from build123d import *

# Parameters (mm, degrees)
CYLINDER008_R     = 5.5
CYLINDER008_DEPTH = 20
CYLINDER009_R     = 1.4
CYLINDER009_DEPTH = 20
BOX002_W          = 16
BOX002_H          = 32
BOX002_DEPTH      = 13
FILLET008_R       = 7
FILLET009_R       = 6
FILLET010_R       = 1
FILLET011_R       = 1
CHAMFER007_SIZE   = 1


with BuildPart() as cylinder:
    # Cylinder008 → Cylinder008 (new body)
    with BuildSketch(Plane.XY):
        Circle(CYLINDER008_R)
    extrude(amount=CYLINDER008_DEPTH)


with BuildPart() as fusion004:
    # Cylinder009 → Cylinder009 (new body)
    with BuildSketch(Plane(origin=(-10, 18, 6.5), x_dir=(0, 0, -1), z_dir=(1, 0, 0))):
        Circle(CYLINDER009_R)
    extrude(amount=CYLINDER009_DEPTH)

    # Fusion004: union Cylinder
    add(cylinder.part)


with BuildPart() as obj1:
    # Box002 → Box002 (new body)
    with BuildSketch(Plane(origin=(-8, -8, 0), x_dir=(1, 0, 0), z_dir=(0, 0, 1))):
        with Locations((8, 16)):
            Rectangle(BOX002_W, BOX002_H)
    extrude(amount=BOX002_DEPTH)

    # Fillet008
    fillet008_edges = [obj1.edges().sort_by_distance(p)[0] for p in [
        (-8, -8, 6.5),
        (8, -8, 6.5),
    ]]
    fillet(fillet008_edges, radius=FILLET008_R)

    # Fillet009
    fillet009_edges = [obj1.edges().sort_by_distance(p)[0] for p in [
        (0, 24, 13),
        (0, 24, 0),
    ]]
    fillet(fillet009_edges, radius=FILLET009_R)

    # Fillet010
    fillet010_edges = [obj1.edges().sort_by_distance(p)[0] for p in [
        (8, 8.5, 13),
    ]]
    fillet(fillet010_edges, radius=FILLET010_R)

    # Cut004: cut Fusion004
    add(fusion004.part, mode=Mode.SUBTRACT)

    # Fillet011
    fillet011_edges = [obj1.edges().sort_by_distance(p)[0] for p in [
        (-5.5, 0, 0),
        (-5.5, 0, 13),
    ]]
    fillet(fillet011_edges, radius=FILLET011_R)

    # Chamfer007
    chamfer007_edges = [obj1.edges().sort_by_distance(p)[0] for p in [
        (-8, 18, 7.9),
        (8, 18, 7.9),
    ]]
    chamfer(chamfer007_edges, length=CHAMFER007_SIZE)


solid = obj1.part
Input: part model. Units: mm. Frame: model coordinates. Round coordinates to 2 decimals unless told otherwise and drop trailing zeros. Order: outer loops, then holes, each group sorted by start corner. A loop starts at its lowest first (then second) coordinate and runs counter-clockwise, first axis right, second up.
1. Mould query, pull axis Z, two halves, no side actions, for faces 1 (the face through (0, 11, 0)), 2 (the face through (0.098, 22.289, 11.196)), 3 (the face through (-0.098, 16.633, 6.803)). Classes: released by +Z, released by -Z, zero draft, split by the parting line, or undercut.
The answers:
face 1: released by -Z
face 2: released by +Z
face 3: undercut
2. Pin query (flat end, axial travel): P1, Ø6, axis at x = -5.5, z = 5.5, coming from the -Y side; P2, Ø2, axis at x = 2.5, z = 8.5, coming from the -Y side; P3, Ø1.5, axis at x = -6.5, z = 3, coming from the +Y side. Return the tip coordinate at first contact, or that it passes through.
The answers:
P1: stops at y = -7.84
P2: stops at y = -7.98
P3: stops at y = 23.56
3. Cut plane B-B, the plane z = 6.5. Output: boundary loops of the cut face in (x, y).
The answers:
outline: (-8, -1) arc R7 ccw to (-1, -8) - (1, -8) arc R7 ccw to (8, -1) - (8, 15.6) - (7, 16.6) - (-7, 16.6) - (-8, 15.6) - close; (-8, 20.4) - (-7, 19.4) - (7, 19.4) - (8, 20.4) - (8, 23) arc R1 ccw to (7, 24) - (-7, 24) arc R1 ccw to (-8, 23) - close; hole circle Ø11 at (0, 0)
4. Cut plane A-A, the plane x = 0. Output: boundary loops of the cut face in (y, z).
The answers:
outline: (-8, 1) arc R1 ccw to (-7, 0) - (-6.5, 0) arc R1 ccw to (-5.5, 1) - (-5.5, 12) arc R1 ccw to (-6.5, 13) - (-7, 13) arc R1 ccw to (-8, 12) - close; (5.5, 1) arc R1 ccw to (6.5, 0) - (18, 0) arc R6 ccw to (24, 6) - (24, 7) arc R6 ccw to (18, 13) - (6.5, 13) arc R1 ccw to (5.5, 12) - close; hole circle Ø2.8 at (18, 6.5)
5. Cut plane C-C, the plane y = 0. Output: boundary loops of the cut face in (x, z), then the cut area to 3 significant figures.
The answers:
outline: (-8, 1) arc R1 ccw to (-7, 0) - (-6.5, 0) arc R1 ccw to (-5.5, 1) - (-5.5, 12) arc R1 ccw to (-6.5, 13) - (-7, 13) arc R1 ccw to (-8, 12) - close; (5.5, 1) arc R1 ccw to (6.5, 0) - (7, 0) arc R1 ccw to (8, 1) - (8, 12) arc R1 ccw to (7, 13) - (6.5, 13) arc R1 ccw to (5.5, 12) - close
area: 63.3 mm2
6. Material intervals for line 1 (Z direction, x = -2, y = 18); line 2 (Y direction, x = 0, z = 7.25); line 3 (X direction, y = 0, z = 4.75), sorted ascending.
The answers:
line 1: z = 0 to 5.1, 7.9 to 13
line 2: y = -8 to -5.5, 5.5 to 16.82, 19.18 to 23.99
line 3: x = -8 to -5.5, 5.5 to 8
